Autodesk Inventor part; units mm, degrees
ref_plane "YZ Plane" through (0, 0, 0) normal (1, 0, 0) x (0, 1, 0)
ref_plane "XZ Plane" through (0, 0, 0) normal (0, 1, 0) x (-1, 0, 0)
ref_plane "XY Plane" through (0, 0, 0) normal (0, 0, 1) x (1, 0, 0)
sketch "스케치1" plane through (0, 0, 0) normal (0, 1, 0) x (-1, 0, 0)
  circle A0 centre (0, 0) radius 51.635
  circle A1 centre (0, 0) radius 53.4089
  dimension "d0" = 103.27
extrude "돌출1" add sketch "스케치1" along normal blind 25
extrude "돌출2" add sketch "스케치1" along normal blind 15 contours A0
sketch "스케치2" plane through (0, 25, 0) normal (0, 1, 0) x (1, 0, 0)
  line L0 (-7, 38.0484) -> (-7, 59.2742)
  line L1 (7, 38.0484) -> (7, 59.2742)
  circle A0 centre (0, 0) radius 53.4089
  circle A1 centre (0, 0) radius 51.635
  point P0 (-7, 51.1583)
  point P1 (7, 51.1583)
  point P2 (7, 52.9482)
  point P3 (-7, 52.9482)
  dimension "d5" = 14
  dimension "d6" = 7
extrude "돌출3" cut sketch "스케치2" against normal blind 10 contours L0 A0 L1 A1 picked at (5.4466, 51.8962)
sketch "스케치5" plane through (0, 0, 0) normal (0, -1, 0) x (1, 0, 0)
  circle A0 centre (0, 0) radius 53.4089
  line L0 (0, 53.4089) -> (0, -53.4089) construction
  line L1 (-53.4089, 0) -> (53.4089, 0) construction
  line L2 (-49.5229, 20) -> (49.5229, 20) construction
  line L3 (49.5229, 20) -> (49.5229, -20) construction
  line L4 (49.5229, -20) -> (-49.5229, -20) construction
  line L5 (-49.5229, -20) -> (-49.5229, 20) construction
  line L6 (-20, 20) -> (20, 20)
  line L7 (20, 20) -> (20, 30)
  line L8 (20, 30) -> (-20, 30)
  line L9 (-20, 30) -> (-20, 20)
  line L10 (20, -20) -> (20, -30)
  line L11 (20, -30) -> (-20, -30)
  line L12 (-20, -30) -> (-20, -20)
  line L13 (-20, -20) -> (20, -20)
  point P0 (0, 30)
  dimension "d19" = 40
  dimension "d20" = 20
  dimension "d21" = 40
  dimension "d22" = 10
extrude "돌출6" add sketch "스케치5" along normal blind 40 contours L9 L8 L7 L6 | L10 L11 L12 L13
sketch "스케치6" plane through (-20, 0, 30) normal (0, 0, 1) x (1, 0, 0)
  line L0 (0, 0) -> (40, 0)
  line L1 (0, 0) -> (0, -40)
  line L2 (40, -40) -> (0, -40)
  line L3 (40, 0) -> (40, -40)
  circle A0 centre (20, -20.074) radius 4
  point P0 (20, 0)
  dimension "d25" = 8
  dimension "d26" = 20.074
  dimension "d27" = 20
extrude "돌출7" cut sketch "스케치6" against normal blind 69.75 contours A0
properties part number "lidar_case"
Could you check a few things on this model? Use its own coordinates, in mm. A direction names the side the tool comes from. Round coordinates to 2 decimals unless told otherwise and drop trailing zeros. Write each loop counter-clockwise with the first axis right and the second up, starting at its lowest first coordinate (ties: lowest second). Pieces come first, ordered by that corner, then holes. Notation, with made-up numbers: M 49,53 L 100,53 A36 ccw 100,92 Z; hole C -38,-32 d3. An arc over 180 degrees is marked long. Write each question's results on one line, items separated by ' | '. Start each with the question number.
1. I'm going to push flat-ended pins straight in: pin 1 Ø12 at (x, y) = (-2.5, -21.5) entering from -Z; pin 2 Ø5 at (x, z) = (-16.5, -41) entering from -Y; pin 3 Ø13 at (x, y) = (0, -20.074) entering from +Z. Where does each tip first touch, or does it pass through?
2. Thinking about a two-plate mould opening in Z: for faces 6 (the face through (-4.2, -19.7, 30)), 7 (the face through (11.58, 12.32, 52.14)), 8 (the face through (4.2, -19.7, 20)), 9 (the face through (-0.87, -23.98, -24.93)), which applies, +Z half, -Z half, draft (parallel to the pull), parting line (faces both ways), or undercut?
3. Imagine slicing it at D-D on x = 33. List the corners of the cut face in (y, z) for me.
4. Imagine slicing it at A-A on x = 0. List the corners of the cut face in (y, z) for me (3 decimals).
5. I need wall thicknesses on L1, parallel to Y at x = 0, z = -26.25; L2, parallel to X at y = 18.75, z = 0 (3 decimals); L3, parallel to Z at x = -3.5, y = -26. Which ranges of each line are inside material? Lowest first, please. Write a range as from..to.
6. Imagine slicing it at B-B on z = 0. List the corners of the cut face in (x, y) for me (3 decimals).
7. Imagine slicing it at C-C on z = -25.5. List the corners of the cut face in (x, y) for me.
8. On a 3-axis mill with a long thin cutter (end or side, diameter ignored), from which of +Z, -Z, +X, -X, +Y, -Y can I reach the whole of each face in a straight line? I mean faces 1 (the face through (-20, -20, 25)), 2 (the face through (4.2, -19.7, -20)), 3 (the face through (-4.2, -19.7, -30)), 4 (the face through (-1, 15, -2)), 5 (the face through (20, -20, 25)). Say none if no direction works.
Result sheet:
1) pin 1: stops at z = -30 | pin 2: stops at y = 0 | pin 3: stops at z = 30
2) face 6: +Z half | face 7: parting line | face 8: undercut | face 9: draft
3) outline: M 0,-41.99 L 25,-41.99 L 25,-39.71 L 15,-39.71 L 15,39.71 L 25,39.71 L 25,41.99 L 0,41.99 Z
4) outline: M -40,-30 L -24.074,-30 L -24.074,-20 L -40,-20 Z; M -40,20 L -24.074,20 L -24.074,30 L -40,30 Z; M -16.074,-30 L 0,-30 L 0,-53.409 L 15,-53.409 L 15,51.635 L 25,51.635 L 25,53.409 L 0,53.409 L 0,30 L -16.074,30 L -16.074,20 L 0,20 L 0,-20 L -16.074,-20 Z
5) L1: y = -40..-24.07, -16.07..15 | L2: x = -53.409..-51.635, 51.635..53.409 | L3: z = -30..-20, 20..30
6) outline: M -53.409,0 L 53.409,0 L 53.409,25 L 51.635,25 L 51.635,15 L -51.635,15 L -51.635,25 L -53.409,25 Z
7) outline: M -46.93,0 L -20,0 L -20,-40 L 20,-40 L 20,0 L 46.93,0 L 46.93,25 L 44.9,25 L 44.9,15 L -44.9,15 L -44.9,25 L -46.93,25 Z; hole C 0,-20.07 d8
8) face 1: +Z, -Z, -X, -Y | face 2: +X, -X, -Y | face 3: -Z, +X, -X, -Y | face 4: +Y | face 5: +Z, -Z, +X, -Y
